Autodesk Inventor part; units mm, degrees
ref_plane "YZ Plane" through (0, 0, 0) normal (1, 0, 0) x (0, 1, 0)
ref_plane "XZ Plane" through (0, 0, 0) normal (0, 1, 0) x (-1, 0, 0)
ref_plane "XY Plane" through (0, 0, 0) normal (0, 0, 1) x (1, 0, 0)
sketch "Sketch1" plane through (0, 0, 0) normal (1, 0, 0) x (0, 1, 0)
  circle A0 centre (0, 0) radius 57.5
  dimension "d0" = 115
extrude "Extrusion1" add sketch "Sketch1" along normal blind 2
sketch "Sketch2" plane through (2, 0, 0) normal (1, 0, 0) x (0, 0, -1)
  circle A0 centre (0, 0) radius 58.5
  dimension "d3" = 117
extrude "Extrusion2" add sketch "Sketch2" along normal blind 1
sketch "Sketch3" plane through (0, 0, 0) normal (-1, 0, 0) x (0, 0, 1)
  circle A0 centre (0, 0) radius 58.5
extrude "Extrusion3" add sketch "Sketch3" along normal blind 1
sketch "Sketch4" plane through (-1, 0, 0) normal (-1, 0, 0) x (0, 0, 1)
  circle A0 centre (0, 0) radius 54
  dimension "d8" = 108
extrude "Extrusion4" cut sketch "Sketch4" against normal blind 5
sketch "Sketch5" plane through (-1, 0, 0) normal (-1, 0, 0) x (0, 0, 1)
  circle A0 centre (0, 0) radius 1.5
  circle A1 centre (0, 0) radius 3.5
  dimension "d11" = 3
  dimension "d12" = 7
extrude "Extrusion5" add sketch "Sketch5" against normal blind 5
sketch "Sketch6" plane through (-1, 0, 0) normal (-1, 0, 0) x (0, 0, 1)
  line L0 (2.7345, 0) -> (2.7345, 2) construction
  line L1 (2.7345, 2) -> (2.7345, -2) construction
  line L2 (2.7345, -2) -> (54.8201, -2)
  line L3 (54.8201, -2) -> (54.8201, 2)
  line L4 (54.8201, 2) -> (2.7345, 2)
  line L5 (2.7345, 2) -> (2.7345, -2)
  point P0 (0, 0)
  dimension "d15" = 2
  dimension "d16" = 4
extrude "Extrusion6" add sketch "Sketch6" against normal blind 4
pattern_circular "Circular Pattern1" count 4 over 360 about axis through (-1, 0, 0) along (1, 0, 0) of "Extrusion6"
sketch "Sketch7" plane through (-1, 0, 0) normal (-1, 0, 0) x (0, 0, 1)
  circle A0 centre (0, 0) radius 1.5
  circle A1 centre (0, 0) radius 4
  dimension "d22" = 8
extrude "Extrusion7" add sketch "Sketch7" against normal blind 15
sketch "Sketch8" plane through (14, 0, 0) normal (1, 0, 0) x (0, 0, -1)
  circle A0 centre (0, 0) radius 1.625
  dimension "d25" = 3.25
extrude "Extrusion8" cut sketch "Sketch8" against normal blind 100
properties part number "mtv_pushingWheel_1-13"
Could you check a few things on this model? Use its own coordinates, in mm. A direction names the side the tool comes from. Give positions to 0.01 mm unless a question says otherwise; leave off trailing zeros. Order: outer loops, then holes, each group sorted by start corner. A loop starts at its lowest first (then second) coordinate and runs counter-clockwise, first axis right, second up. Notation, with made-up numbers: (29, -11) -> (60, -11) arc R7 ccw to (60, -7) -> close; hole circle Ø8 at (17, 29). An arc over 180 degrees is marked (long way). Return JSON: item names as keys, results as strings.
1. On a 3-axis mill with a long thin cutter (end or side, diameter ignored), from which of +Z, -Z, +X, -X, +Y, -Y can I reach the whole of each face in a straight line? I mean faces 1 (the cylindrical face through (8.06, 2.7, -2.95)), 2 (the flat face through (1, -2, 28)), 3 (the flat face through (2, -39, -43)), 4 (the flat face through (-1, 0, 4)). Say none if no direction works.
Answer list:
{"face 1": "+X", "face 2": "+X, -X", "face 3": "none", "face 4": "+Z, -Z, -X, +Y, -Y"}
2. I need wall thicknesses on line 1 (Y direction, x = 5.25, z = 0) (3 decimals); line 2 (Z direction, x = 1, y = 46.5); line 3 (Z direction, x = 1.5, y = 28.5). Which ranges of each line are inside material? Lowest first, please. Write a range as from..to.
Answer list:
{"line 1": "y = -4..-1.625, 1.625..4", "line 2": "z = -33.82..-27.45, -2..2, 27.45..33.82", "line 3": "z = -49.94..-45.87, -2..2, 45.87..49.94"}
3. Imagine slicing it at C-C on y = 34.5. List the corners of the cut face in (x, z) for me.
Answer list:
{"outline": "(-1, -47.24) -> (0, -47.24) -> (0, -46) -> (2, -46) -> (2, -47.24) -> (3, -47.24) -> (3, -41.54) -> (-1, -41.54) -> close; (-1, -2) -> (3, -2) -> (3, 2) -> (-1, 2) -> close; (-1, 41.54) -> (3, 41.54) -> (3, 47.24) -> (2, 47.24) -> (2, 46) -> (0, 46) -> (0, 47.24) -> (-1, 47.24) -> close"}
4. Thinking about a two-plate mould opening in Y: for faces 5 (the flat face through (14, 0, 2)), 6 (the cylindrical face through (0.972, 37.782, 38.582)), 7 (the cylindrical face through (-0.49, 57.11, -12.68)), which applies, pulls with the +Y half, pulls with the -Y half, needs draft (parallel to the pull), parting line crosses it, or undercut?
Answer list:
{"face 5": "needs draft", "face 6": "undercut", "face 7": "parting line crosses it"}
5. For pin 1 Ø4 at (y, z) = (-46, -34.5) entering from +X; pin 2 Ø4.5 at (x, y) = (0, 39) entering from -Z; pin 3 Ø1.2 at (x, y) = (1.5, -22.5) entering from +Z, each with a flat end and sliding along its axis, tell me the tip position at first contact or that it passes through.
Answer list:
{"pin 1": "stops at x = 3", "pin 2": "stops at z = -45.52", "pin 3": "stops at z = 54.14"}
6. Imagine slicing it at A-A on z = 0. List the corners of the cut face in (x, y) for me (3 decimals).
Answer list:
{"outline": "(-1, -58.5) -> (0, -58.5) -> (0, -57.5) -> (2, -57.5) -> (2, -58.5) -> (3, -58.5) -> (3, -4) -> (14, -4) -> (14, -1.625) -> (-1, -1.625) -> close; (-1, 1.625) -> (14, 1.625) -> (14, 4) -> (3, 4) -> (3, 58.5) -> (2, 58.5) -> (2, 57.5) -> (0, 57.5) -> (0, 58.5) -> (-1, 58.5) -> close"}
7. Imagine slicing it at D-D on x = 7. List the corners of the cut face in (y, z) for me (3 decimals), then the cut area to 3 significant figures.
Answer list:
{"outline": "circle Ø8 at (0, 0); hole circle Ø3.25 at (0, 0)", "area": "42.0 mm2"}
